from build123d import *
from build123d.topology import SkipClean

# Parameters (mm, degrees)
SKETCH3_R          = 12.7
CUT_EXTRUDE1_DEPTH = 48.768
CUT_EXTRUDE2_DEPTH = 19.05


with BuildPart() as part:
    # Sketch1 → Revolve1 (revolve)
    with BuildSketch(Plane.XY, mode=Mode.PRIVATE) as revolve1_sk:
        Polygon((0, 0), (12.7, 0), (12.7, 3.175), (53.975, 3.175), (53.975, 79.375), (41.275, 79.375), (41.275, 53.975), (15.875, 53.975), (15.875, 22.225), (0, 22.225), align=None)
    revolve(revolve1_sk.sketch.rotate(Axis((0, 22.225, 0), (0, -1, 0)), 180), axis=Axis((0, 22.225, 0), (0, -1, 0)))

    # Sketch3 → Cut-Extrude1 (cut)
    with BuildSketch(Plane(origin=(0, 0, -53.975), x_dir=(-1, 0, 0), z_dir=(0, 0, -1))):
        with Locations((0, 34.925)):
            Circle(SKETCH3_R)
    extrude(amount=-CUT_EXTRUDE1_DEPTH, mode=Mode.SUBTRACT)

    # Sketch4 → Cut-Extrude2 (cut)
    with SkipClean():  # the faces are left unmerged after this step: merging them gives an invalid solid
        with BuildSketch(Plane(origin=(0, 53.975, 0), x_dir=(1, 0, 0), z_dir=(0, 1, 0))):
            with BuildLine():
                Line((-12.7, 15.875), (-12.7, 0))
                Line((-12.7, 0), (12.7, 0))
                Line((12.7, 0), (12.7, 15.875))
                ThreePointArc((12.7, 15.875), (0, 28.575), (-12.7, 15.875))
            make_face()
        extrude(amount=-CUT_EXTRUDE2_DEPTH, mode=Mode.SUBTRACT)


solid = part.part
For this review, take the finished solid that the model builds, in its own axes (mm). A direction names the side the tool comes from. Give positions to 0.01 mm unless a question says otherwise; leave off trailing zeros. Loops run counter-clockwise (first coordinate to the right, second up) from the corner with the lowest first, then second, coordinate; pieces in that order, holes last. Notation, with made-up numbers: (0, 50) -> (52, 50) arc R9 ccw to (52, 59) -> close; hole circle Ø3 at (57, 67.25). An arc over 180 degrees is marked (long way). One line per question, with ' | ' between items.
1) We need section B-B (x = 28.5). Write out the cut boundary in (y, z) (3 decimals), plus the area to 3 significant figures.
Resolved:
outline: (3.175, -45.837) -> (79.375, -45.837) -> (79.375, -29.856) -> (53.975, -29.856) -> (53.975, 29.856) -> (79.375, 29.856) -> (79.375, 45.837) -> (3.175, 45.837) -> close | area: 5,470 mm2
2) The part is to be moulded in two halves that separate along X. For faces 4 (the flat face through (12, 79.375, 40)), 5 (the cylindrical face through (-5.86, 1.61, 11.267)), 6 (the flat face through (-12.7, 45, -13)), say which applies: +X half, -X half, draft (parallel to the pull), parting line (faces both ways), or undercut.
Resolved:
face 4: draft | face 5: parting line | face 6: undercut
3) For faces 1 (the flat face through (0, 0, 0)), 2 (the cylindrical face through (5.373, 66.497, -40.924)), 3 (the cylindrical face through (2.753, 22.527, -37)), list the 3-axis set-ups (+Z, -Z, +X, -X, +Y, -Y) from which the entire face can be reached by the end or side of a thin tool; tool diameter is ignored.
Resolved:
face 1: +Z, -Z, +X, -X, -Y | face 2: +Y | face 3: -Z
4) We need section D-D (y = 38). Write out the cut boundary in (x, z) (3 decimals).
Resolved:
outline: (-12.7, -15.875) -> (-12.7, -9.525) arc R15.875 cw (long way) to (12.7, -9.525) -> (12.7, -15.875) arc R12.7 cw to (12.322, -18.95) -> (12.322, -52.55) arc R53.975 ccw (long way) to (-12.322, -52.55) -> (-12.322, -18.95) arc R12.7 cw to start
5) Insertion check: pin 1 Ø1 at (x, y) = (16.5, 51) entering from -Z; pin 2 Ø3 at (x, y) = (-43, 36.5) entering from -Z; pin 3 Ø6 at (x, z) = (-35.5, -26.5) entering from -Y (3 decimals). Each pin has a flat end and moves straight along its axis. Give the tip position at first contact, or say it passes through.
Resolved:
pin 1: stops at z = -51.55 | pin 2: stops at z = -34.51 | pin 3: stops at y = 3.175
6) To check wall thickness, follow probe 1 along Y at (x, z) = (-46.5, 0.5) (3 decimals); probe 2 along Y at (x, z) = (-19.5, 10.5) (3 decimals); probe 3 along Z at (x, y) = (-10.5, 44). State the ranges of each line that lie inside material, in increasing order.
Resolved:
probe 1: y = 3.175 to 79.375 | probe 2: y = 3.175 to 53.975 | probe 3: z = -52.94 to -23.02, 11.91 to 52.94
7) We need section A-A (z = -30.5). Write out the cut boundary in (x, y) (3 decimals).
Resolved:
outline: (-44.531, 3.175) -> (44.531, 3.175) -> (44.531, 79.375) -> (27.81, 79.375) -> (27.81, 53.975) -> (-27.81, 53.975) -> (-27.81, 79.375) -> (-44.531, 79.375) -> close; hole circle Ø25.4 at (0, 34.925)
8) We need section C-C (z = -19). Write out the cut boundary in (x, y) (3 decimals).
Resolved:
outline: (-50.52, 3.175) -> (50.52, 3.175) -> (50.52, 79.375) -> (36.642, 79.375) -> (36.642, 53.975) -> (12.31, 53.975) -> (12.31, 38.05) arc R12.7 cw (long way) to (-12.31, 38.05) -> (-12.31, 53.975) -> (-36.642, 53.975) -> (-36.642, 79.375) -> (-50.52, 79.375) -> close
